Source: three-view drawing plus pictorial views. Frame: mm from the lowest corner of the part. Give positions to 0.01 mm unless a question says otherwise; leave off trailing zeros. Order: outer loops, then holes, each group sorted by start corner. A loop starts at its lowest first (then second) coordinate and runs counter-clockwise, first axis right, second up. Notation, with made-up numbers: M 28,80 L 56,80 A23 cw 56,96 Z; hole C 77,73 d6. An arc over 180 degrees is marked long. One line per item, written item: value. Start each with the question number.
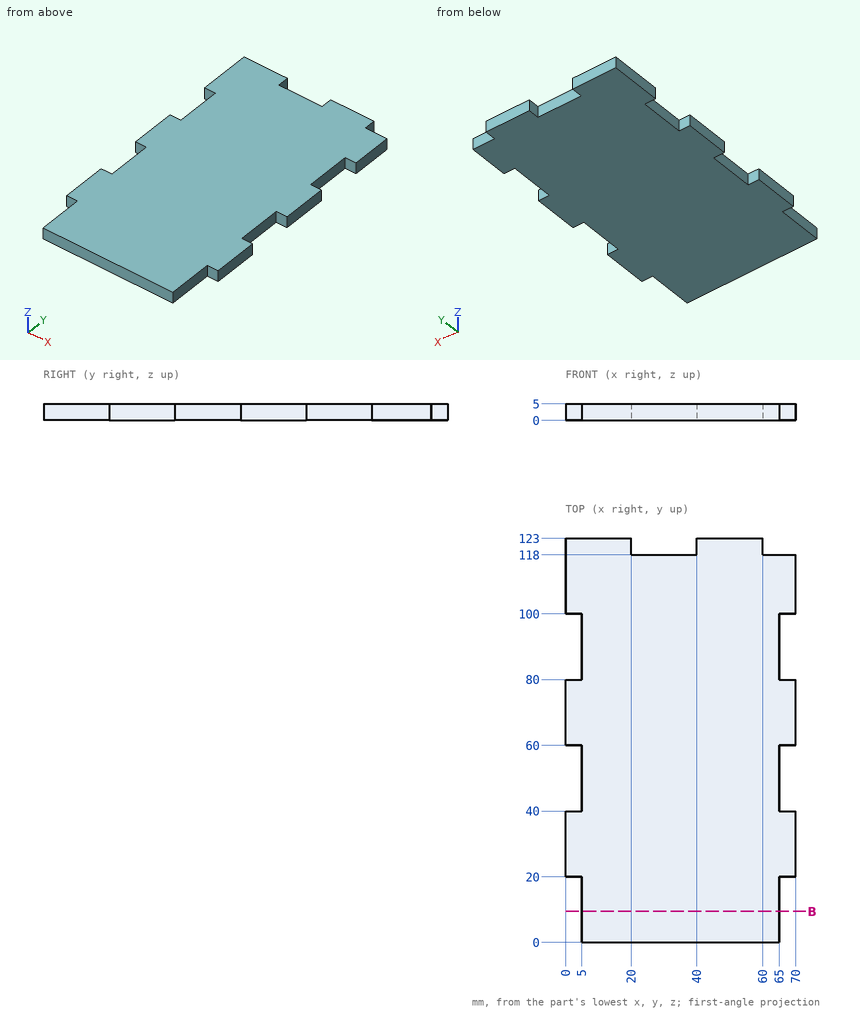
Q1. Section query B-B on y = 9.5. Return loops of the section in (x, z), and give its area (3 significant figures).
Q2. Contact query for flat-ended pins moving along their axis: pin 1 (2 mm diameter, centred on y = 58.5, z = 3, fed in from +X); pin 2 (2.5 mm diameter, centred on x = 1.5, z = 3.5, fed in from -Y); pin 3 (2.5 mm diameter, centred on y = 49.5, z = 2.5, fed in from -X). Output: stop coordinate, or through.
Q3. Ray query, line 1 along Y through (x, z) = (28, 0.35); line 2 along X through (y, z) = (58, 2). Return the intervals inside material, ascending. Write a range as [from, to].
Results below:
1. outline: M 5,0 L 65,0 L 65,5 L 5,5 Z
1. area: 300 mm2
2. pin 1: x = 65
2. pin 2: y = 20
2. pin 3: x = 5
3. line 1: [0, 118]
3. line 2: [5, 65]
